For this review, take the finished solid that the model builds, in its own axes (mm). A direction names the side the tool comes from. Give positions to 0.01 mm unless a question says otherwise; leave off trailing zeros. Loops run counter-clockwise (first coordinate to the right, second up) from the corner with the lowest first, then second, coordinate; pieces in that order, holes last. Notation, with made-up numbers: (51, 29.5) - (69, 29.5) arc R29 ccw to (69, 58.5) - close; hole circle Ø9 at (18, 15.25). An arc over 180 degrees is marked (long way). Put each result on its own line as item: value.
from build123d import *

# Parameters (mm, degrees)
SKETCH_1_W          = 26
SKETCH_1_H          = 29
EXTRUDE_1_DEPTH     = 6
SKETCH_2_R          = 1.25
CUT_EXTRUDE_1_DEPTH = 21.377683872
SKETCH_4_W          = 16
SKETCH_4_H          = 23
CUT_EXTRUDE_3_DEPTH = 2
CUT_EXTRUDE_4_DEPTH = 1.5
FILLET_1_R          = 1
SKETCH_6_R          = 1.95
CUT_EXTRUDE_5_DEPTH = 1
FILLET_3_R          = 3
SKETCH_8_W          = 6
SKETCH_8_H          = 21
CUT_EXTRUDE_6_DEPTH = 3.5
FILLET_2_R          = 1
FILLET_4_R          = 1
CUT_EXTRUDE_7_REACH = 30.675
SKETCH_9_W          = 6
SKETCH_9_H          = 8
FILLET_5_R          = 3
CHAMFER_2_SIZE      = 1


# Some blends are built 0.0001 mm under size
with BuildPart() as part:
    # Эскиз1 → Бобышка-Вытянуть1 (new body)
    with BuildSketch(Plane(origin=(0, 0, 0), x_dir=(0, 0, -1), z_dir=(1, 0, 0))):
        Rectangle(SKETCH_1_W, SKETCH_1_H)
    extrude(amount=EXTRUDE_1_DEPTH)

    # Эскиз2 → Вырез-Вытянуть1 (cut, through all)
    with BuildSketch(Plane.ZY):
        with Locations((-7, 7.75)):
            Circle(SKETCH_2_R)
        with Locations((-7, -7.75)):
            Circle(SKETCH_2_R)
    extrude(amount=-CUT_EXTRUDE_1_DEPTH, mode=Mode.SUBTRACT)

    # Эскиз4 → Вырез-Вытянуть3 (cut)
    with BuildSketch(Plane.ZY):
        with Locations((-3, 0)):
            Rectangle(SKETCH_4_W, SKETCH_4_H)
    extrude(amount=-CUT_EXTRUDE_3_DEPTH, mode=Mode.SUBTRACT)

    # Эскиз5 → Вырез-Вытянуть4 (cut)
    with BuildSketch(Plane.ZY.offset(-2)):
        Polygon((-11, -3.5), (-11, 3.5), (-6, 3.5), (-6, 10.5), (5, 10.5), (5, -10.5), (-6, -10.5), (-6, -3.5), align=None)
    extrude(amount=-CUT_EXTRUDE_4_DEPTH, mode=Mode.SUBTRACT)

    # Скругление1
    fillet_1_edges = [part.edges().sort_by_distance(p)[0] for p in [
        (2.75, 7, -6),
        (2.75, 3.5, -6),
        (2.75, 8.5, -6),
        (2.75, -8.5, -6),
        (2.75, -7, -6),
        (2.75, 3.5, -11),
        (2.75, -3.5, -6),
        (2.75, -3.5, -11),
    ]]
    fillet(fillet_1_edges, radius=FILLET_1_R)

    # Эскиз6 → Вырез-Вытянуть5 (cut)
    with BuildSketch(Plane(origin=(6, 0, 0), x_dir=(0, 0, -1), z_dir=(1, 0, 0))):
        with Locations((7, 7.75)):
            Circle(SKETCH_6_R)
        with Locations((7, -7.75)):
            Circle(SKETCH_6_R)
    extrude(amount=-CUT_EXTRUDE_5_DEPTH, mode=Mode.SUBTRACT)

    # Скругление3
    fillet_3_edges = [part.edges().sort_by_distance(p)[0] for p in [
        (6, 0, 13),
        (6, 0, -13),
    ]]
    fillet(fillet_3_edges, radius=FILLET_3_R)

    # Эскиз8 → Вырез-Вытянуть6 (cut)
    with BuildSketch(Plane.ZY):
        with Locations((8, 0)):
            Rectangle(SKETCH_8_W, SKETCH_8_H)
    extrude(amount=-CUT_EXTRUDE_6_DEPTH, mode=Mode.SUBTRACT)

    # Скругление2
    fillet_2_edges = [part.edges().sort_by_distance(p)[0] for p in [
        (1, -11.5, -11),
        (1, -11.5, 5),
        (2.75, -10.5, -6),
        (1, 11.5, -11),
        (1, 11.5, 5),
        (2.75, 10.5, -6),
        (1.75, -10.5, 11),
        (1.75, 10.5, 11),
    ]]
    fillet(fillet_2_edges, radius=FILLET_2_R - 0.0001)  # a hair under: the kernel refuses the full size

    # Скругление4
    # the kernel refuses this fillet: 1 mm, written as the material it takes off along each edge
    with BuildSketch(Plane(origin=(-1.830232679, -10.5, 5), x_dir=(0, 0, 1), z_dir=(1, 0, 0))) as fillet_4_piece_1:
        with BuildLine():
            CenterArc((0.732093072, 1), FILLET_4_R, 209.998345944, 60.001654056)
            Line((-0.133946766, 0.500025001), (-0.22055075, 0.450027501))
            ThreePointArc((-0.22055075, 0.450027501), (-0.1, 0.0001), (-0.1, 0))
            Line((-0.1, 0), (0, -0.1))
            Line((0, -0.1), (0.732093072, -0.1))
            Line((0.732093072, -0.1), (0.732093072, 0))
        make_face()
    extrude(amount=3.830232679, mode=Mode.SUBTRACT)
    with BuildSketch(Plane(origin=(-1.830232679, 10.5, 5), x_dir=(0, 0, 1), z_dir=(1, 0, 0))) as fillet_4_piece_2:
        with BuildLine():
            CenterArc((0.732093072, -1), FILLET_4_R, 90, 60.001654056)
            Line((-0.133946766, -0.500025001), (-0.22055075, -0.450027501))
            ThreePointArc((-0.22055075, -0.450027501), (-0.1, -0.0001), (-0.1, 0))
            Line((-0.1, 0), (0, 0.1))
            Line((0, 0.1), (0.732093072, 0.1))
            Line((0.732093072, 0.1), (0.732093072, 0))
        make_face()
    extrude(amount=3.830232679, mode=Mode.SUBTRACT)

    # Эскиз9 → Вырез-Вытянуть7 (cut, up to next)
    with BuildSketch(Plane(origin=(0, 0, 11), x_dir=(-1, 0, 0), z_dir=(0, 0, -1)), mode=Mode.PRIVATE) as cut_extrude_7_sk1:
        Rectangle(SKETCH_9_W, SKETCH_9_H)
    cut_extrude_7_tool1 = extrude(cut_extrude_7_sk1.sketch, amount=-CUT_EXTRUDE_7_REACH, mode=Mode.PRIVATE) & part.part
    add(cut_extrude_7_tool1.solids().sort_by_distance((0, 0, 11))[0], mode=Mode.SUBTRACT)

    # Скругление5
    fillet_5_edges = [part.edges().sort_by_distance(p)[0] for p in [
        (3, -4, 12),
        (3, 4, 12),
    ]]
    fillet(fillet_5_edges, radius=FILLET_5_R - 0.0001)  # a hair under: the kernel refuses the full size

    # Фаска2
    chamfer_2_edges = [part.edges().sort_by_distance(p)[0] for p in [
        (6, 14.5, 0),
        (6, -14.5, 0),
        (1.5, -14.5, -13),
        (1.5, -14.5, 13),
        (5.121320344, -14.5, -12.121320344),
        (5.121320344, -14.5, 12.121320344),
        (1.5, 14.5, 13),
        (1.5, 14.5, -13),
        (5.121320344, 14.5, -12.121320344),
        (5.121320344, 14.5, 12.121320344),
    ]]
    chamfer(chamfer_2_edges, length=CHAMFER_2_SIZE)


solid = part.part
1) Draft analysis for pull direction Z (two halves, no side actions). For faces 1 (the face through (2.14, 3.1, 12.01)), 2 (the face through (2.74, -6.215, -6.301)), 3 (the face through (1, 9, 13)), state which applies: pulls with the +Z half, pulls with the -Z half, needs draft (parallel to the pull), parting line crosses it, or undercut.
Geometry check:
face 1: needs draft
face 2: undercut
face 3: pulls with the +Z half
2) Wall thickness on line 1 (Y direction, x = 3.25, z = -7); line 2 (Y direction, x = 3.75, z = -7); line 3 (Y direction, x = 5.5, z = -6.75): over which ranges is each line inside the solid? List them lowest first.
Geometry check:
line 1: y = -14.5 to -9, -6.5 to -3.5, 3.5 to 6.5, 9 to 14.5
line 2: y = -14.5 to -9, -6.5 to 6.5, 9 to 14.5
line 3: y = -14 to -9.68, -5.82 to 5.82, 9.68 to 14
3) For faces 4 (the face through (4.666, 14.118, 11.703)), 5 (the face through (2.1, -3.14, 12.01)), 6 (the face through (1, 11.5, -3)), list the 3-axis set-ups (+Z, -Z, +X, -X, +Y, -Y) from which the entire face can be reached by the end or side of a thin tool; tool diameter is ignored.
Geometry check:
face 4: +Z, +X, +Y
face 5: +Z, -X
face 6: -X
4) Take a section at C-C on y = -5. State the section outline as (x, z) points.
Geometry check:
outline: (0, -13) - (3, -13) arc R3 ccw to (6, -10) - (6, 10) arc R3 ccw to (3, 13) - (0, 13) - (0, 11) - (3.5, 11) - (3.5, -6) - (2, -6) - (2, -11) - (0, -11) - close
5) Take a section at B-B on z = 1.25. State the section outline as (x, y) points.
Geometry check:
outline: (0, -14.5) - (5, -14.5) - (6, -13.5) - (6, 13.5) - (5, 14.5) - (0, 14.5) - (0, 11.5) - (2, 11.5) - (2, 10.5) - (3.5, 10.5) - (3.5, -10.5) - (2, -10.5) - (2, -11.5) - (0, -11.5) - close
6) Insertion check: pin 1 Ø2.5 at (y, z) = (-8, -1) entering from -X; pin 2 Ø3 at (y, z) = (-7.75, -7) entering from -X; pin 3 Ø1.9 at (y, z) = (7, -7) entering from +X. Each pin has a flat end and moves straight along its axis. Give the tip position at first contact, or say it passes through.
Geometry check:
pin 1: stops at x = 3.5
pin 2: stops at x = 2
pin 3: stops at x = 5
7) Take a section at D-D on x = 1. State the section outline as (y, z) points.
Geometry check:
outline: (-14.5, -12) - (-13.5, -13) - (13.5, -13) - (14.5, -12) - (14.5, 12) - (13.5, 13) - (3.83, 13) - (3.83, 11) - (9.5, 11) arc R1 cw to (10.5, 10) - (10.5, 5.73) arc R1 ccw to (11, 4.87) arc R1 cw to (11.5, 4) - (11.5, -10) arc R1 cw to (10.5, -11) - (-10.5, -11) arc R1 cw to (-11.5, -10) - (-11.5, 4) arc R1 cw to (-11, 4.87) arc R1 ccw to (-10.5, 5.73) - (-10.5, 10) arc R1 cw to (-9.5, 11) - (-3.83, 11) - (-3.83, 13) - (-13.5, 13) - (-14.5, 12) - close
8) Take a section at A-A on y = 7.75. State the section outline as (x, z) points, and give its area (3 significant figures).
Geometry check:
outline: (0, -13) - (3, -13) arc R3 ccw to (6, -10) - (6, -8.95) - (5, -8.95) - (5, -8.25) - (2, -8.25) - (2, -11) - (0, -11) - close; (0, 11) - (3.5, 11) - (3.5, -5.75) - (5, -5.75) - (5, -5.05) - (6, -5.05) - (6, 10) arc R3 ccw to (3, 13) - (0, 13) - close
area: 71.6 mm²
